Design review of the part built by this model. Coordinates are the model's own, in mm. A direction names the side the tool comes from. Coordinates: 2 decimals unless noted, no trailing zeros. Loops run counter-clockwise (first coordinate to the right, second up) from the corner with the lowest first, then second, coordinate; pieces in that order, holes last.
Q1. For P1, Ø12, axis at x = 50.5, z = -59.5, coming from the +Y side, flat-tipped, find the tip position at first contact; note if it passes through.
Q2. Draft analysis for pull direction Z (two halves, no side actions). For faces 1 (the face through (78.757, 3.042, 69.871)), 2 (the face through (-2, 0, -16)), state which applies: released by +Z, released by -Z, zero draft, split by the parting line, or undercut.
Q3. Machinability: for faces 3 (the face through (-78.757, 3.042, -97.871)), 4 (the face through (-2, 6, -16)), which of the approach directions +Z, -Z, +X, -X, +Y, -Y give a long, thin tool a straight path to every point of the face, cutting with its end or side? Answer none if there is none.
Q4. Wall thickness on probe 1 along X at (y, z) = (1.9, -178); probe 2 along Z at (x, y) = (-12, 3.5); probe 3 along Z at (x, y) = (-125.5, 4.75): over which ranges is each line inside the solid? List them lowest first.
Q5. Add section C-C on z = -98.5. Give the boundary of the cut face in (x, y).
Q6. Add section A-A on x = -68. Give the boundary of the cut face in (y, z).
Q7. Add section B-B on y = 2. Give the number of separate pieces and of enclosed holes in the cut face, and give its area (3 significant figures).
```python
from build123d import *

# Parameters (mm, degrees)
SKETCH_1_R            = 1.65
EXTRUDE_1_DEPTH       = 6
SKETCH_3_R            = 2.1
SKETCH_3_W            = 7
SKETCH_3_H            = 6
CUT_EXTRUDE_1_DEPTH   = 7
SKETCH_31_R           = 2.1
SKETCH_31_W           = 7
SKETCH_31_H           = 6
CUT_EXTRUDE_11_DEPTH  = 7
SKETCH_32_R           = 2.1
SKETCH_32_W           = 7
SKETCH_32_H           = 6
CUT_EXTRUDE_12_DEPTH  = 7
SKETCH_33_R           = 2.1
SKETCH_33_W           = 7
SKETCH_33_H           = 6
CUT_EXTRUDE_13_DEPTH  = 7
SKETCH_34_R           = 2.1
SKETCH_34_W           = 7
SKETCH_34_H           = 6
CUT_EXTRUDE_14_DEPTH  = 7
SKETCH_35_R           = 2.1
SKETCH_35_W           = 7
SKETCH_35_H           = 6
CUT_EXTRUDE_15_DEPTH  = 7
SKETCH_37_R           = 2.1
SKETCH_37_W           = 7
SKETCH_37_H           = 6
CUT_EXTRUDE_17_DEPTH  = 7
SKETCH_38_R           = 2.1
SKETCH_38_W           = 7
SKETCH_38_H           = 6
CUT_EXTRUDE_18_DEPTH  = 7
SKETCH_39_R           = 2.1
SKETCH_39_W           = 7
SKETCH_39_H           = 6
CUT_EXTRUDE_19_DEPTH  = 7
SKETCH_310_R          = 2.1
SKETCH_310_W          = 7
SKETCH_310_H          = 6
CUT_EXTRUDE_110_DEPTH = 7
SKETCH_311_R          = 2.1
SKETCH_311_W          = 7
SKETCH_311_H          = 6
CUT_EXTRUDE_111_DEPTH = 7
SKETCH_312_R          = 2.1
SKETCH_312_W          = 7
SKETCH_312_H          = 6
CUT_EXTRUDE_112_DEPTH = 7
CUT_EXTRUDE_113_DEPTH = 7


with BuildPart() as part:
    # Эскиз1 → Бобышка-Вытянуть1 (new body)
    with BuildSketch(Plane(origin=(0, 0, 0), x_dir=(1, 0, 0), z_dir=(0, 1, 0))):
        with BuildLine():
            Line((-154, -156), (154, -156))
            ThreePointArc((154, -156), (158.242640687, -154.242640687), (160, -150))
            Line((160, -150), (160, 178))
            ThreePointArc((160, 178), (158.242640687, 182.242640687), (154, 184))
            Line((154, 184), (-154, 184))
            ThreePointArc((-154, 184), (-158.242640687, 182.242640687), (-160, 178))
            Line((-160, 178), (-160, -150))
            ThreePointArc((-160, -150), (-158.242640687, -154.242640687), (-154, -156))
        make_face()
        with Locations((-154, 178)):
            Circle(SKETCH_1_R, mode=Mode.SUBTRACT)
        with Locations((154, 178)):
            Circle(SKETCH_1_R, mode=Mode.SUBTRACT)
        with Locations((-154, -150)):
            Circle(SKETCH_1_R, mode=Mode.SUBTRACT)
        with Locations((154, -150)):
            Circle(SKETCH_1_R, mode=Mode.SUBTRACT)
    extrude(amount=EXTRUDE_1_DEPTH)

    # Эскиз3 → Вырез-Вытянуть1 (cut, through all)
    with BuildSketch(Plane(origin=(-23, 6, 20), x_dir=(1, 0, 0), z_dir=(0, 1, 0))):
        with Locations((0, 47)):
            Circle(SKETCH_3_R)
        with Locations((9.531849908, 47)):
            Rectangle(SKETCH_3_W, SKETCH_3_H)
        with Locations((-9.531849908, 47)):
            Rectangle(SKETCH_3_W, SKETCH_3_H)
    extrude(amount=-CUT_EXTRUDE_1_DEPTH, mode=Mode.SUBTRACT)

    # Эскиз31 → Вырез-Вытянуть11 (cut, through all)
    with BuildSketch(Plane(origin=(-23, 6, -48), x_dir=(-1, 0, 0), z_dir=(0, 1, 0))):
        with Locations((0, 47)):
            Circle(SKETCH_31_R)
        with Locations((9.531849908, 47)):
            Rectangle(SKETCH_31_W, SKETCH_31_H)
        with Locations((-9.531849908, 47)):
            Rectangle(SKETCH_31_W, SKETCH_31_H)
    extrude(amount=-CUT_EXTRUDE_11_DEPTH, mode=Mode.SUBTRACT)

    # Эскиз32 → Вырез-Вытянуть12 (cut, through all)
    with BuildSketch(Plane(origin=(23, 6, 20), x_dir=(1, 0, 0), z_dir=(0, 1, 0))):
        with Locations((0, 47)):
            Circle(SKETCH_32_R)
        with Locations((9.531849908, 47)):
            Rectangle(SKETCH_32_W, SKETCH_32_H)
        with Locations((-9.531849908, 47)):
            Rectangle(SKETCH_32_W, SKETCH_32_H)
    extrude(amount=-CUT_EXTRUDE_12_DEPTH, mode=Mode.SUBTRACT)

    # Эскиз33 → Вырез-Вытянуть13 (cut, through all)
    with BuildSketch(Plane(origin=(23, 6, -48), x_dir=(-1, 0, 0), z_dir=(0, 1, 0))):
        with Locations((0, 47)):
            Circle(SKETCH_33_R)
        with Locations((9.531849908, 47)):
            Rectangle(SKETCH_33_W, SKETCH_33_H)
        with Locations((-9.531849908, 47)):
            Rectangle(SKETCH_33_W, SKETCH_33_H)
    extrude(amount=-CUT_EXTRUDE_13_DEPTH, mode=Mode.SUBTRACT)

    # Эскиз34 → Вырез-Вытянуть14 (cut, through all)
    with BuildSketch(Plane(origin=(43.5, 6, 72.7), x_dir=(-1, 0, 0), z_dir=(0, 1, 0))):
        with Locations((0, 47)):
            Circle(SKETCH_34_R)
        with Locations((9.531849908, 47)):
            Rectangle(SKETCH_34_W, SKETCH_34_H)
        with Locations((-9.531849908, 47)):
            Rectangle(SKETCH_34_W, SKETCH_34_H)
    extrude(amount=-CUT_EXTRUDE_14_DEPTH, mode=Mode.SUBTRACT)

    # Эскиз35 → Вырез-Вытянуть15 (cut, through all)
    with BuildSketch(Plane(origin=(43.5, 6, 139.3), x_dir=(1, 0, 0), z_dir=(0, 1, 0))):
        with Locations((0, 47)):
            Circle(SKETCH_35_R)
        with Locations((9.531849908, 47)):
            Rectangle(SKETCH_35_W, SKETCH_35_H)
        with Locations((-9.531849908, 47)):
            Rectangle(SKETCH_35_W, SKETCH_35_H)
    extrude(amount=-CUT_EXTRUDE_15_DEPTH, mode=Mode.SUBTRACT)

    # Эскиз37 → Вырез-Вытянуть17 (cut, through all)
    with BuildSketch(Plane(origin=(-43.5, 6, 139.3), x_dir=(1, 0, 0), z_dir=(0, 1, 0))):
        with Locations((0, 47)):
            Circle(SKETCH_37_R)
        with Locations((9.531849908, 47)):
            Rectangle(SKETCH_37_W, SKETCH_37_H)
        with Locations((-9.531849908, 47)):
            Rectangle(SKETCH_37_W, SKETCH_37_H)
    extrude(amount=-CUT_EXTRUDE_17_DEPTH, mode=Mode.SUBTRACT)

    # Эскиз38 → Вырез-Вытянуть18 (cut, through all)
    with BuildSketch(Plane(origin=(-43.5, 6, 72.7), x_dir=(-1, 0, 0), z_dir=(0, 1, 0))):
        with Locations((0, 47)):
            Circle(SKETCH_38_R)
        with Locations((9.531849908, 47)):
            Rectangle(SKETCH_38_W, SKETCH_38_H)
        with Locations((-9.531849908, 47)):
            Rectangle(SKETCH_38_W, SKETCH_38_H)
    extrude(amount=-CUT_EXTRUDE_18_DEPTH, mode=Mode.SUBTRACT)

    # Эскиз39 → Вырез-Вытянуть19 (cut, through all)
    with BuildSketch(Plane(origin=(-43.5, 6, -100.7), x_dir=(1, 0, 0), z_dir=(0, 1, 0))):
        with Locations((0, 47)):
            Circle(SKETCH_39_R)
        with Locations((9.531849908, 47)):
            Rectangle(SKETCH_39_W, SKETCH_39_H)
        with Locations((-9.531849908, 47)):
            Rectangle(SKETCH_39_W, SKETCH_39_H)
    extrude(amount=-CUT_EXTRUDE_19_DEPTH, mode=Mode.SUBTRACT)

    # Эскиз310 → Вырез-Вытянуть110 (cut, through all)
    with BuildSketch(Plane(origin=(43.5, 6, -100.7), x_dir=(1, 0, 0), z_dir=(0, 1, 0))):
        with Locations((0, 47)):
            Circle(SKETCH_310_R)
        with Locations((9.531849908, 47)):
            Rectangle(SKETCH_310_W, SKETCH_310_H)
        with Locations((-9.531849908, 47)):
            Rectangle(SKETCH_310_W, SKETCH_310_H)
    extrude(amount=-CUT_EXTRUDE_110_DEPTH, mode=Mode.SUBTRACT)

    # Эскиз311 → Вырез-Вытянуть111 (cut, through all)
    with BuildSketch(Plane(origin=(-43.5, 6, -167.3), x_dir=(-1, 0, 0), z_dir=(0, 1, 0))):
        with Locations((0, 47)):
            Circle(SKETCH_311_R)
        with Locations((9.531849908, 47)):
            Rectangle(SKETCH_311_W, SKETCH_311_H)
        with Locations((-9.531849908, 47)):
            Rectangle(SKETCH_311_W, SKETCH_311_H)
    extrude(amount=-CUT_EXTRUDE_111_DEPTH, mode=Mode.SUBTRACT)

    # Эскиз312 → Вырез-Вытянуть112 (cut, through all)
    with BuildSketch(Plane(origin=(43.5, 6, -167.3), x_dir=(-1, 0, 0), z_dir=(0, 1, 0))):
        with Locations((0, 47)):
            Circle(SKETCH_312_R)
        with Locations((9.531849908, 47)):
            Rectangle(SKETCH_312_W, SKETCH_312_H)
        with Locations((-9.531849908, 47)):
            Rectangle(SKETCH_312_W, SKETCH_312_H)
    extrude(amount=-CUT_EXTRUDE_112_DEPTH, mode=Mode.SUBTRACT)

    # Эскиз313 → Вырез-Вытянуть113 (cut, through all)
    with BuildSketch(Plane(origin=(0, 6, 0), x_dir=(1, 0, 0), z_dir=(0, 1, 0))):
        with BuildLine():
            Line((-127.516979969, 144.745730497), (-127.516979969, 49.590777688))
            ThreePointArc((-127.516979969, 49.590777688), (-126.931193532, 48.176564126), (-125.516979969, 47.590777688))
            Line((-125.516979969, 47.590777688), (-36.16415843, 47.590777688))
            ThreePointArc((-36.16415843, 47.590777688), (-34.328657222, 48.796463318), (-34.706193444, 50.959842369))
            Line((-34.706193444, 50.959842369), (-124.059014984, 146.114795178))
            ThreePointArc((-124.059014984, 146.114795178), (-126.253210242, 146.605290925), (-127.516979969, 144.745730497))
        make_face()
        with BuildLine():
            Line((34.706193444, 50.959842369), (124.059014984, 146.114795178))
            ThreePointArc((124.059014984, 146.114795178), (126.253210242, 146.605290925), (127.516979969, 144.745730497))
            Line((127.516979969, 144.745730497), (127.516979969, 49.590777688))
            ThreePointArc((127.516979969, 49.590777688), (126.931193532, 48.176564126), (125.516979969, 47.590777688))
            Line((125.516979969, 47.590777688), (36.16415843, 47.590777688))
            ThreePointArc((36.16415843, 47.590777688), (34.328657222, 48.796463318), (34.706193444, 50.959842369))
        make_face()
        with BuildLine():
            Line((127.516979969, -116.745730497), (127.516979969, -21.590777688))
            ThreePointArc((127.516979969, -21.590777688), (126.931193532, -20.176564126), (125.516979969, -19.590777688))
            Line((125.516979969, -19.590777688), (36.16415843, -19.590777688))
            ThreePointArc((36.16415843, -19.590777688), (34.328657222, -20.796463318), (34.706193444, -22.959842369))
            Line((34.706193444, -22.959842369), (124.059014984, -118.114795178))
            ThreePointArc((124.059014984, -118.114795178), (126.253210242, -118.605290925), (127.516979969, -116.745730497))
        make_face()
        with BuildLine():
            Line((-34.706193444, -22.959842369), (-124.059014984, -118.114795178))
            ThreePointArc((-124.059014984, -118.114795178), (-126.253210242, -118.605290925), (-127.516979969, -116.745730497))
            Line((-127.516979969, -116.745730497), (-127.516979969, -21.590777688))
            ThreePointArc((-127.516979969, -21.590777688), (-126.931193532, -20.176564126), (-125.516979969, -19.590777688))
            Line((-125.516979969, -19.590777688), (-36.16415843, -19.590777688))
            ThreePointArc((-36.16415843, -19.590777688), (-34.328657222, -20.796463318), (-34.706193444, -22.959842369))
        make_face()
    extrude(amount=-CUT_EXTRUDE_113_DEPTH, mode=Mode.SUBTRACT)


solid = part.part
```
Entries:
1. P1: stops at y = 6
2. face 1: undercut
2. face 2: zero draft
3. face 3: +Y, -Y
3. face 4: +Z, -Z, +X, -X, +Y
4. probe 1: x = -160 to -155.65, -152.35 to 152.35, 155.65 to 160
4. probe 2: z = -184 to -30, -24 to -4, 2 to 156
4. probe 3: z = -184 to -146.75, -47.59 to 19.59, 118.75 to 156
5. outline: (-160, 0) - (-127.52, 0) - (-127.52, 6) - (-160, 6) - close; (-79.35, 0) - (79.35, 0) - (79.35, 6) - (-79.35, 6) - close; (127.52, 0) - (160, 0) - (160, 6) - (127.52, 6) - close
6. outline: (0, -184) - (6, -184) - (6, -86.42) - (0, -86.42) - close; (0, -47.59) - (6, -47.59) - (6, 19.59) - (0, 19.59) - close; (0, 58.42) - (6, 58.42) - (6, 156) - (0, 156) - close
7. separate pieces: 1
7. enclosed holes: 44
7. area: 88,000 mm2
